Model file for the job. Use its own axes, mm. A direction names the side the tool comes from. Round coordinates to 2 decimals unless told otherwise and drop trailing zeros. Loops run counter-clockwise (first coordinate to the right, second up) from the corner with the lowest first, then second, coordinate; pieces in that order, holes last. Notation, with made-up numbers: M 84.25,5.5 L 96.25,5.5 A18 ccw 96.25,17.5 Z; hole C 3.25,-4.75 d1. An arc over 180 degrees is marked long. Answer in a Markdown table with one row per item.
from build123d import *
from build123d.topology import SkipClean

# Parameters (mm, degrees)
BOSS_EXTRUDE1_DEPTH      = 4
SKETCH1_W                = 0.8
SKETCH1_H                = 0.35
BOSS_EXTRUDE1_2_DEPTH    = 4
BOSS_EXTRUDE1_3_DEPTH    = 4
BOSS_EXTRUDE1_4_DEPTH    = 4
BOSS_EXTRUDE1_5_DEPTH    = 4
SKETCH2_W                = 0.6
SKETCH2_H                = 0.35
SKETCH2_W_2              = 0.8
SKETCH2_W_3              = 2
BOSS_EXTRUDE2_DEPTH      = 1.5
SKETCH3_W                = 2
SKETCH3_H                = 0.5
BOSS_EXTRUDE3_DEPTH      = 1.5
BOSS_EXTRUDE4_DEPTH      = 3.7
BOSS_EXTRUDE6_DEPTH      = 3.2
BOSS_EXTRUDE7_REACH      = 33.958
BOSS_EXTRUDE7_END_RADIUS = 11
SKETCH7_W                = 3
SKETCH7_H                = 0.4
BOSS_EXTRUDE8_REACH      = 33.958
SKETCH8_W                = 3
SKETCH8_H                = 0.4
SKETCH9_R                = 1
BOSS_EXTRUDE9_DEPTH      = 2
SKETCH5_R                = 8.5
BOSS_EXTRUDE5_DEPTH      = 4.952033783
FILLET1_R                = 0.25
FILLET2_R                = 0.25
SKETCH10_R               = 5.5
CUT_EXTRUDE1_DEPTH       = 2
CUT_EXTRUDE2_DEPTH       = 29.992852085
BOSS_EXTRUDE10_START     = -8.652034
BOSS_EXTRUDE10_DEPTH     = 8.652034
CIRPATTERN2_COUNT        = 4
SKETCH13_R               = 6.95
SKETCH13_R_2             = 5.95
CUT_EXTRUDE3_DEPTH       = 4.952033783
CHAMFER1_SIZE            = 1
CUT_EXTRUDE4_REACH       = 35.954
CUT_EXTRUDE4_END_RADIUS  = 6.95
CUT_EXTRUDE5_START       = -17
CUT_EXTRUDE5_DEPTH       = 2.01521
CUT_EXTRUDE6_START       = -2.000004
SKETCH16_R               = 8.5
CUT_EXTRUDE6_DEPTH       = 2.000004


with BuildPart() as part:
    # Sketch1 → Boss-Extrude1 (new body)
    with BuildSketch(Plane(origin=(0, 0, 0), x_dir=(1, 0, 0), z_dir=(0, 1, 0))):
        Polygon((9.796794919, 19.233012702), (10.143205081, 19.433012702), (10.643205081, 18.566987298), (10.296794919, 18.366987298), align=None)
    extrude(amount=BOSS_EXTRUDE1_DEPTH)



with BuildPart() as body_2:
    # Sketch1 → Boss-Extrude1 2 (new body)
    with BuildSketch(Plane(origin=(0, 0, 0), x_dir=(1, 0, 0), z_dir=(0, 1, 0))):
        with Locations((-3, 0)):
            Rectangle(SKETCH1_W, SKETCH1_H)
    extrude(amount=BOSS_EXTRUDE1_2_DEPTH)


with BuildPart() as body_3:
    # Sketch1 → Boss-Extrude1 3 (new body)
    with BuildSketch(Plane(origin=(0, 0, 0), x_dir=(1, 0, 0), z_dir=(0, 1, 0))):
        Rectangle(SKETCH1_W, SKETCH1_H)
    extrude(amount=BOSS_EXTRUDE1_3_DEPTH)


with BuildPart() as body_4:
    # Sketch1 → Boss-Extrude1 4 (new body)
    with BuildSketch(Plane(origin=(0, 0, 0), x_dir=(1, 0, 0), z_dir=(0, 1, 0))):
        with Locations((3, 0)):
            Rectangle(SKETCH1_W, SKETCH1_H)
    extrude(amount=BOSS_EXTRUDE1_4_DEPTH)


with BuildPart() as body_5:
    # Sketch1 → Boss-Extrude1 5 (new body)
    with BuildSketch(Plane(origin=(0, 0, 0), x_dir=(1, 0, 0), z_dir=(0, 1, 0))):
        Polygon((-10.296794919, 18.366987298), (-10.643205081, 18.566987298), (-10.143205081, 19.433012702), (-9.796794919, 19.233012702), align=None)
    extrude(amount=BOSS_EXTRUDE1_5_DEPTH)


with BuildPart() as part_1:
    add(part.part)

    add(body_2.part)  # Boss-Extrude2 merges body 2

    add(body_3.part)  # Boss-Extrude2 merges body 3

    add(body_4.part)  # Boss-Extrude2 merges body 4

    add(body_5.part)  # Boss-Extrude2 merges body 5
    # Sketch2 → Boss-Extrude2 (add)
    with BuildSketch(Plane(origin=(0, 4, 0), x_dir=(1, 0, 0), z_dir=(0, 1, 0))):
        Polygon((-11.143205081, 17.700961894), (-9.643205081, 20.299038106), (-9.296794919, 20.099038106), (-10.796794919, 17.500961894), align=None)
        Polygon((9.643205081, 20.299038106), (11.143205081, 17.700961894), (10.796794919, 17.500961894), (9.296794919, 20.099038106), align=None)
        with Locations((0.7, 0)):
            Rectangle(SKETCH2_W, SKETCH2_H)
        Rectangle(SKETCH2_W_2, SKETCH2_H)
        with Locations((-0.7, 0)):
            Rectangle(SKETCH2_W, SKETCH2_H)
        with Locations((-3, 0)):
            Rectangle(SKETCH2_W_3, SKETCH2_H)
        with Locations((3, 0)):
            Rectangle(SKETCH2_W_3, SKETCH2_H)
    extrude(amount=BOSS_EXTRUDE2_DEPTH)

    # Sketch3 → Boss-Extrude3 (add)
    with BuildSketch(Plane(origin=(0, 0, -0.175), x_dir=(-1, 0, 0), z_dir=(0, 0, -1))):
        with Locations((-3, 5.25)):
            Rectangle(SKETCH3_W, SKETCH3_H)
        with Locations((0, 5.25)):
            Rectangle(SKETCH3_W, SKETCH3_H)
        with Locations((3, 5.25)):
            Rectangle(SKETCH3_W, SKETCH3_H)
    extrude(amount=BOSS_EXTRUDE3_DEPTH)

    # Sketch4 → Boss-Extrude4 (add)
    with BuildSketch(Plane.XZ.offset(-5)):
        with BuildLine():
            Line((-4.75, -1.675), (4.75, -1.675))
            Line((4.75, -1.675), (4.75, -3.175))
            ThreePointArc((4.75, -3.175), (0, -24.096567416), (-4.75, -3.175))
            Line((-4.75, -3.175), (-4.75, -1.675))
        make_face()
    extrude(amount=-BOSS_EXTRUDE4_DEPTH)

    # Sketch6 → Boss-Extrude6 (add)
    with BuildSketch(Plane(origin=(0, 5.5, 0), x_dir=(1, 0, 0), z_dir=(0, 1, 0))):
        Polygon((-9.643205081, 20.299038106), (-11.143205081, 17.700961894), (-10.796794919, 17.500961894), (-9.296794919, 20.099038106), align=None)
        Polygon((11.143205081, 17.700961894), (9.643205081, 20.299038106), (9.296794919, 20.099038106), (10.796794919, 17.500961894), align=None)
    extrude(amount=BOSS_EXTRUDE6_DEPTH)

    # Boss-Extrude7: up to this cylinder (the profile starts outside it)
    boss_extrude7_end = Plane(origin=(0, 8.5, -13.096567416), z_dir=(0, -1, 0)) * Cylinder(BOSS_EXTRUDE7_END_RADIUS, 90.916, mode=Mode.PRIVATE)
    # Sketch7 → Boss-Extrude7 (add, up to the surface)
    with BuildSketch(Plane(origin=(15.675734985, 0, -9.050389813), x_dir=(0.4999999999999947, 0, 0.8660254037844417), z_dir=(-0.8660254037844418, 0, 0.49999999999999484)), mode=Mode.PRIVATE) as boss_extrude7_sk1:
        with Locations((-11.257880132, 8.5)):
            Rectangle(SKETCH7_W, SKETCH7_H)
    boss_extrude7_tool1 = extrude(boss_extrude7_sk1.sketch, amount=BOSS_EXTRUDE7_REACH, mode=Mode.PRIVATE) - boss_extrude7_end
    add(boss_extrude7_tool1.solids().sort_by_distance((10.046795, 8.5, -18.8))[0])

    # Sketch8 → Boss-Extrude8 (add, up to next)
    with BuildSketch(Plane(origin=(-15.675734985, 0, -9.050389813), x_dir=(0.4999999999999956, 0, -0.8660254037844413), z_dir=(0.8660254037844413, 0, 0.4999999999999956)), mode=Mode.PRIVATE) as boss_extrude8_sk1:
        with Locations((11.257880132, 8.5)):
            Rectangle(SKETCH8_W, SKETCH8_H)
    boss_extrude8_tool1 = extrude(boss_extrude8_sk1.sketch, amount=BOSS_EXTRUDE8_REACH, mode=Mode.PRIVATE) - part_1.part
    add(boss_extrude8_tool1.solids().sort_by_distance((-10.046795, 8.5, -18.8))[0])

    # Sketch9 → Boss-Extrude9 (add)
    with BuildSketch(Plane.XZ.offset(-5)):
        with Locations(Location((-8.5, -13.096567416, 0), (0, 0, 90))):
            Circle(SKETCH9_R)
        with Locations(Location((8.5, -13.096567416, 0), (0, 0, 90))):
            Circle(SKETCH9_R)
    extrude(amount=BOSS_EXTRUDE9_DEPTH)

    # Sketch5 → Boss-Extrude5 (add)
    with BuildSketch(Plane(origin=(0, 8.7, 0), x_dir=(1, 0, 0), z_dir=(0, 1, 0))):
        with Locations(Location((0, 13.096567416, 0), (0, 0, 270))):
            Circle(SKETCH5_R)
    extrude(amount=BOSS_EXTRUDE5_DEPTH)

    # Fillet1
    fillet1_edges = [part_1.edges().sort_by_distance(p)[0] for p in [
        (-10.393205081, 8.7, -19),
        (-10.046794919, 8.3, -18.8),
        (-3, 5.5, 0.175),
        (-3, 5, -0.175),
        (3, 5, -0.175),
        (0, 5, -0.175),
        (0, 5.5, 0.175),
        (3, 5.5, 0.175),
        (10.046794919, 8.3, -18.8),
        (10.393205081, 8.7, -19),
    ]]
    fillet(fillet1_edges, radius=FILLET1_R)

    # Fillet2
    fillet2_edges = [part_1.edges().sort_by_distance(p)[0] for p in [
        (-3.4, 0, 0),
        (-2.6, 0, 0),
        (-10.47, 0, -18.466987298),
        (-0.4, 0, 0),
        (0.4, 0, 0),
        (2.6, 0, 0),
        (3.4, 0, 0),
        (-9.97, 0, -19.333012702),
        (10.47, 0, -18.466987298),
        (9.97, 0, -19.333012702),
    ]]
    fillet(fillet2_edges, radius=FILLET2_R)

    # Sketch10 → Cut-Extrude1 (cut)
    with BuildSketch(Plane(origin=(0, 13.652033783, 0), x_dir=(1, 0, 0), z_dir=(0, 1, 0))):
        with Locations(Location((0, 13.096567416, 0), (0, 0, 270))):
            Circle(SKETCH10_R)
    extrude(amount=-CUT_EXTRUDE1_DEPTH, mode=Mode.SUBTRACT)

    # Sketch11 → Cut-Extrude2 (cut, through all)
    with BuildSketch(Plane(origin=(0, 11.652033783, 0), x_dir=(1, 0, 0), z_dir=(0, 1, 0))):
        with BuildLine():
            Line((-5.319305603, 14.494776234), (-1.398208818, 18.41587302))
            ThreePointArc((-1.398208818, 18.41587302), (-0.952383252, 18.513482234), (-0.5, 18.573792992))
            Line((-0.5, 18.573792992), (-0.5, 17.446567416))
            Line((-0.5, 17.446567416), (0.5, 17.446567416))
            Line((0.5, 17.446567416), (0.5, 18.573792992))
            ThreePointArc((0.5, 18.573792992), (0.952383252, 18.513482234), (1.398208818, 18.41587302))
            Line((1.398208818, 18.41587302), (5.319305603, 14.494776234))
            ThreePointArc((5.319305603, 14.494776234), (5.5, 13.096567416), (5.319305603, 11.698358599))
            Line((5.319305603, 11.698358599), (1.398208818, 7.777261813))
            ThreePointArc((1.398208818, 7.777261813), (0.952383252, 7.679652599), (0.5, 7.619341841))
            Line((0.5, 7.619341841), (0.5, 8.746567416))
            Line((0.5, 8.746567416), (-0.5, 8.746567416))
            Line((-0.5, 8.746567416), (-0.5, 7.619341841))
            ThreePointArc((-0.5, 7.619341841), (-0.952383252, 7.679652599), (-1.398208818, 7.777261813))
            Line((-1.398208818, 7.777261813), (-5.319305603, 11.698358599))
            ThreePointArc((-5.319305603, 11.698358599), (-5.5, 13.096567416), (-5.319305603, 14.494776234))
        make_face()
    extrude(amount=-CUT_EXTRUDE2_DEPTH, mode=Mode.SUBTRACT)

    # Sketch12 → Boss-Extrude10 (add)
    with BuildSketch(Plane(origin=(0, 13.652033783, 0), x_dir=(1, 0, 0), z_dir=(0, 1, 0)).offset(BOSS_EXTRUDE10_START)):
        with BuildLine():
            Line((-2.208630624, 18.133625165), (-1.803122292, 17.728116833))
            Line((-1.803122292, 17.728116833), (-1.032444553, 18.498794573))
            ThreePointArc((-1.032444553, 18.498794573), (-1.630790989, 18.349235381), (-2.208630624, 18.133625165))
        make_face()
        with BuildLine():
            Line((-5.037057749, 15.305198041), (-4.631549417, 14.899689709))
            Line((-4.631549417, 14.899689709), (-5.402227156, 14.129011969))
            ThreePointArc((-5.402227156, 14.129011969), (-5.252667965, 14.727358405), (-5.037057749, 15.305198041))
        make_face()
    boss_extrude10 = extrude(amount=BOSS_EXTRUDE10_DEPTH)

    # CirPattern2: Boss-Extrude10 ×4 about axis
    cirpattern2_axis = Axis((0, 0, -13.096567416), (0, 1, 0))
    for i in range(1, CIRPATTERN2_COUNT):
        add(boss_extrude10.rotate(cirpattern2_axis, i * 360 / CIRPATTERN2_COUNT))

    # Sketch13 → Cut-Extrude3 (cut)
    with SkipClean():  # the faces are left unmerged after this step: merging them gives an invalid solid
        with BuildSketch(Plane(origin=(0, 13.652033783, 0), x_dir=(1, 0, 0), z_dir=(0, 1, 0))):
            with Locations(Location((0, 13.096567416, 0), (0, 0, 270))):
                Circle(SKETCH13_R)
            with Locations(Location((0, 13.096567416, 0), (0, 0, 270))):
                Circle(SKETCH13_R_2, mode=Mode.SUBTRACT)
        extrude(amount=-CUT_EXTRUDE3_DEPTH, mode=Mode.SUBTRACT)

    # Chamfer1
    chamfer1_edges = [part_1.edges().sort_by_distance(p)[0] for p in [
        (0, 13.652033783, -21.596567416),
    ]]
    chamfer(chamfer1_edges, length=CHAMFER1_SIZE)

    # Cut-Extrude4: up to this cylinder (the profile starts outside it)
    with SkipClean():  # the faces are left unmerged after this step: merging them gives an invalid solid
        cut_extrude4_end = Plane(origin=(0, 12.3187, -13.096567416), z_dir=(0, 1, 0)) * Cylinder(CUT_EXTRUDE4_END_RADIUS, 86.808, mode=Mode.PRIVATE)
        # Sketch14 → Cut-Extrude4 (cut, up to the surface)
        with BuildSketch(Plane(origin=(8.5, 0, 0), x_dir=(0, 0, -1), z_dir=(1, 0, 0)), mode=Mode.PRIVATE) as cut_extrude4_sk1:
            Polygon((10.596567416, 13.652033783), (12.596567416, 11.652033783), (12.596567416, 9.652033783), (13.596567416, 9.652033783), (13.596567416, 11.652033783), (15.596567416, 13.652033783), align=None)
        cut_extrude4_tool1 = extrude(cut_extrude4_sk1.sketch, amount=-CUT_EXTRUDE4_REACH, mode=Mode.PRIVATE) - cut_extrude4_end
        add(cut_extrude4_tool1.solids().sort_by_distance((8.5, 12.3187, -13.096567))[0], mode=Mode.SUBTRACT)

    # Sketch14<2> → Cut-Extrude5 (cut)
    with SkipClean():  # the faces are left unmerged after this step: merging them gives an invalid solid
        with BuildSketch(Plane(origin=(8.5, 0, 0), x_dir=(0, 0, -1), z_dir=(1, 0, 0)).offset(CUT_EXTRUDE5_START)):
            Polygon((10.596567416, 13.652033783), (12.596567416, 11.652033783), (12.596567416, 9.652033783), (13.596567416, 9.652033783), (13.596567416, 11.652033783), (15.596567416, 13.652033783), align=None)
        extrude(amount=CUT_EXTRUDE5_DEPTH, mode=Mode.SUBTRACT)

    # Sketch16 → Cut-Extrude6 (cut)
    with BuildSketch(Plane(origin=(0, 13.652033783, 0), x_dir=(1, 0, 0), z_dir=(0, 1, 0)).offset(CUT_EXTRUDE6_START)):
        with Locations(Location((0, 13.096567416, 0), (0, 0, 3.372286684))):
            Circle(SKETCH16_R)
    extrude(amount=CUT_EXTRUDE6_DEPTH, mode=Mode.SUBTRACT)


solid = part_1.part
1. Saw through at A-A (y = 6.5). State how many separate pieces and enclosed holes the cut face has, and give its area (3 significant figures).
Verdict:
| item | result |
|---|---|
| separate pieces | 3 |
| enclosed holes | 1 |
| area | 310 mm² |
2. Saw through at B-B (z = -6.5). Write the cut outline in (x, y).
Verdict:
| item | result |
|---|---|
| outline | M -8.8,5 L 8.8,5 L 8.8,8.7 L 5.36,8.7 L 5.36,11.65 L 2.19,11.65 L 2.19,8.7 L -2.19,8.7 L -2.19,11.65 L -5.36,11.65 L -5.36,8.7 L -8.8,8.7 Z |
3. Saw through at D-D (z = -2.75). Write the cut outline in (x, y), and give its area (4 significant figures).
Verdict:
| item | result |
|---|---|
| outline | M -4.75,5 L 4.75,5 L 4.75,8.7 L -4.75,8.7 Z |
| area | 35.15 mm² |
4. Tool access for faces 5 (the flat face through (3.339, 8.373, -16.475)), 6 (the flat face through (1, 5, 0)), 7 (the flat face through (-8, 11, -12.597)): list every direction of +Z, -Z, +X, -X, +Y, -Y with a clear straight run to the whole face (end or side of a thin tool).
Verdict:
| item | result |
|---|---|
| face 5 | +Y, -Y |
| face 6 | +Z, +Y, -Y |
| face 7 | -X, +Y |
5. Pin check, flat tips, straight feed: pin 1 (2 mm diameter, centred on x = 2, z = -17.5, fed in from -Y); pin 2 (6 mm diameter, centred on x = 4, y = 9, fed in from +Z) (3 decimals); pin 3 (3 mm diameter, centred on y = 2, z = -19.5, fed in from +X). Stop position of each tip, or through.
Verdict:
| item | result |
|---|---|
| pin 1 | stops at y = 5 |
| pin 2 | stops at z = -1.675 |
| pin 3 | stops at x = 10.64 |
6. Saw through at C-C (x = -8). Write the cut outline in (y, z).
Verdict:
| item | result |
|---|---|
| outline | M 3,-13.96 L 5,-13.96 L 5,-20.65 L 8.7,-20.65 L 8.7,-15.97 L 11.65,-15.97 L 11.65,-13.6 L 9.65,-13.6 L 9.65,-12.6 L 11.65,-12.6 L 11.65,-10.22 L 8.7,-10.22 L 8.7,-5.55 L 5,-5.55 L 5,-12.23 L 3,-12.23 Z |
7. Mould opens along X. For faces 1 (the cylindrical face through (-9.49, 4.01, -13.23)), 2 (the flat face through (-10.38, 5.1, -19.02)), 3 (the cylindrical face through (-5.5, 8.4, -13.1)), 4 (the flat face through (-8, 9.652, -13)) say: +X half, -X half, draft (parallel to the pull), parting line (faces both ways), or undercut.
Verdict:
| item | result |
|---|---|
| face 1 | undercut |
| face 2 | -X half |
| face 3 | undercut |
| face 4 | draft |
8. Wall check: probe 1 along Z at (x, y) = (3.5, 11.25); probe 2 along Y at (x, z) = (6.75, -15.25); probe 3 along Y at (x, z) = (-8.5, -6.75). Give the ranges that are in metal, low to high.
Verdict:
| item | result |
|---|---|
| probe 1 | z = -20.84 to -19.1, -17.91 to -16.31, -9.88 to -8.28, -7.09 to -5.35 |
| probe 2 | y = 5 to 11.65 |
| probe 3 | y = 5 to 8.7 |
